The model under review builds one solid part; all positions refer to its coordinate system, in mm. A direction names the side the tool comes from. Coordinates: 2 decimals unless noted, no trailing zeros. Loops run counter-clockwise (first coordinate to the right, second up) from the corner with the lowest first, then second, coordinate; pieces in that order, holes last. Notation, with made-up numbers: (39, 57.25) - (71, 57.25) arc R21 cw to (71, 77.25) - close; hole circle Ø10 at (55, 51.25). An arc over 180 degrees is marked (long way). Use a Markdown table: item, result. Add a question column.
1) To check wall thickness, follow L1, parallel to Z at x = 32.5, y = -32.5 (3 decimals); L2, parallel to Y at x = 80, z = 53.5; L3, parallel to X at y = -18, z = 4.5 (3 decimals). State the ranges of each line that lie inside material, in increasing order. Write a range as [from, to].
2) Add section B-B, the plane z = 2.5. Give the boundary of the cut face in (x, y) (3 decimals).
3) Clearance check with flat-ended pins moving along their axes: pin 1 (1 mm diameter, centred on x = -2.5, y = 41.5, fed in from +Z) (3 decimals); pin 2 (8 mm diameter, centred on y = -19.5, z = 40.5, fed in from -X); pin 3 (1 mm diameter, centred on x = 28, y = 6.5, fed in from +Z). State where each tip first meets the part, or that it passes through.
4) Add section C-C, the plane x = 77. Give the boundary of the cut face in (y, z).
5) For faces 1 (the cylindrical face through (32.727, -19.139, 51.953)), 2 (the flat face through (46, -25.4, 42)), 3 (the cylindrical face through (32.727, 18.961, 51.953)), 4 (the flat face through (71, 0, 42.862)), list the 3-axis set-ups (+Z, -Z, +X, -X, +Y, -Y) from which the entire face can be reached by the end or side of a thin tool; tool diameter is ignored.
```python
from build123d import *

# Parameters (mm, degrees)
F1_DEPTH = 63.5
F0_W     = 25.4
F0_H     = 19.05
F2_DEPTH = 25.4
F3_DEPTH = 12.7


with BuildPart() as f1:
    # F0 (on Front) → F1 (new body, symmetric)
    with BuildSketch(Plane.XZ):
        Polygon((41.275, -9.525), (41.275, 9.525), (22.225, 9.525), (-41.275, 9.525), (-41.275, -9.525), align=None)
    extrude(amount=F1_DEPTH, both=True)

    # F0 (on Front) → F2 (join, symmetric)
    with BuildSketch(Plane.XZ):
        with BuildLine():
            Line((22.225, 9.525), (41.275, 9.525))
            Line((41.275, 9.525), (41.275, 26.9875))
            ThreePointArc((41.275, 26.9875), (45.9246798487, 38.2128201513), (57.15, 42.8625))
            Line((57.15, 42.8625), (60.325, 42.8625))
            Line((60.325, 42.8625), (60.325, 61.9125))
            Line((60.325, 61.9125), (57.15, 61.9125))
            ThreePointArc((57.15, 61.9125), (32.4542956671, 51.6832043329), (22.225, 26.9875))
            Line((22.225, 26.9875), (22.225, 9.525))
        make_face()
        with Locations((73.025, 52.3875)):
            Rectangle(F0_W, F0_H)
    extrude(amount=F2_DEPTH, both=True)

    # F0 (on Front) → F3 (join, symmetric)
    with BuildSketch(Plane.XZ):
        with BuildLine():
            Line((-41.275, 9.525), (22.225, 9.525))
            Line((22.225, 9.525), (22.225, 26.9875))
            ThreePointArc((22.225, 26.9875), (32.4542956671, 51.6832043329), (57.15, 61.9125))
            add(Edge.make_bspline(
                [(-41.275, 9.525), (-41.275, 36.84458516), (10.5578337313, 61.9125), (57.15, 61.9125)],
                knots=[0, 0, 0, 0, 111.4985685166, 111.4985685166, 111.4985685166, 111.4985685166], degree=3))
        make_face()
    extrude(amount=F3_DEPTH, both=True)


solid = f1.part
```
From the geometry:
| question | item | result |
|---|---|---|
| 1 | L1 | z = [-9.525, 9.525] |
| 1 | L2 | y = [-25.4, 25.4] |
| 1 | L3 | x = [-41.275, 41.275] |
| 2 | outline | (-41.275, -63.5) - (41.275, -63.5) - (41.275, 63.5) - (-41.275, 63.5) - close |
| 3 | pin 1 | stops at z = 9.525 |
| 3 | pin 2 | stops at x = 23.55 |
| 3 | pin 3 | stops at z = 58.98 |
| 4 | outline | (-25.4, 42.86) - (25.4, 42.86) - (25.4, 61.91) - (-25.4, 61.91) - close |
| 5 | face 1 | +Z, -X, -Y |
| 5 | face 2 | +Z, +X, -X, -Y |
| 5 | face 3 | +Z, -X, +Y |
| 5 | face 4 | -Z, +X, +Y, -Y |
